Part model, mm, in its own coordinate system. Face numbers are marked on the shaded views. A direction names the side the tool comes from. Round coordinates to 2 decimals unless told otherwise and drop trailing zeros. Order: outer loops, then holes, each group sorted by start corner. A loop starts at its lowest first (then second) coordinate and runs counter-clockwise, first axis right, second up. Notation, with made-up numbers: (61, 87) -> (71, 87) arc R16 cw to (71, 101) -> close; hole circle Ø7 at (-37, 51.25). An arc over 180 degrees is marked (long way). Return JSON: item names as keys, results as strings. Group by question number.
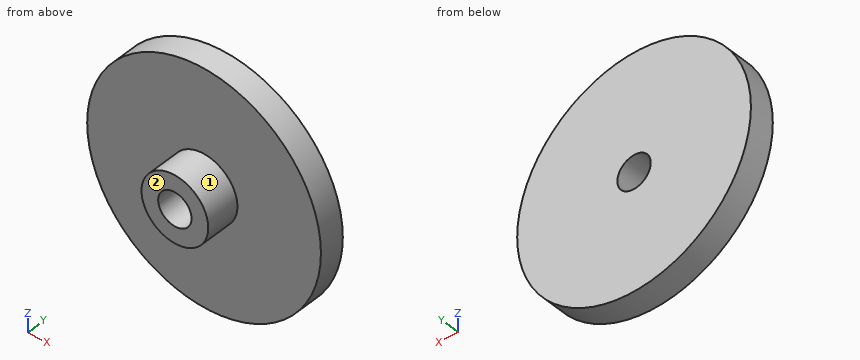
from build123d import *

# Parameters (mm, degrees)
F0_R          = 22.225
F1_DEPTH      = 4.7625
F2_R          = 6.35
F3_DEPTH      = 6.35
F4_R          = 3.175
F5_DEPTH      = 25.4
F5_DEPTH_BACK = 73


# Not quite as in the source:
# - an extrude ends at something that could not be found from the text; its depth is read off the source's solid


with BuildPart() as f1:
    # F0 (on Front) → F1 (new body)
    with BuildSketch(Plane.XZ):
        Circle(F0_R)
    extrude(amount=F1_DEPTH)

    # F2 (on face) → F3 (join)
    with BuildSketch(Plane.XZ.offset(4.7625)):
        Circle(F2_R)
    extrude(amount=F3_DEPTH)

    # F4 (on face) → F5 (cut, two sides)
    with BuildSketch(Plane.XZ.offset(11.1125)) as f5_sk:
        Circle(F4_R)
    extrude(amount=-F5_DEPTH, mode=Mode.SUBTRACT)
    extrude(f5_sk.sketch, amount=F5_DEPTH_BACK, mode=Mode.SUBTRACT)


solid = f1.part
(1) Tool access for the marked faces 1 and 2: list every direction of +Z, -Z, +X, -X, +Y, -Y with a clear straight run to the whole face (end or side of a thin tool).
(2) Saw through at D-D, the plane z = -7.5. List the corners of the cut face in (x, y).
(3) Pin check, flat tips, straight feed: P1, Ø1, axis at x = 4, z = 16, coming from the -Y side; P2, Ø4, axis at x = -14, y = -6.5, coming from the +Z side; P3, Ø2, axis at y = -3.5, z = 15.5, coming from the -X side. Stop position of each tip, or through.
(4) Saw through at C-C, the plane y = -5.5. List the corners of the cut face in (x, z) (3 decimals).
(5) Probe L1, parallel to Z at x = 0, y = -3 (3 decimals); L2, parallel to Z at x = 0, y = -5.25 (3 decimals); L3, parallel to Y at x = 5.5, z = 18. List the from-to ranges inside material, lowest first. Write a range as [from, to].
Results are:
{
 "1": {"face 1": "-Y", "face 2": "+Z, -Z, +X, -X, -Y"},
 "2": {"outline": "(-20.92, -4.76) -> (20.92, -4.76) -> (20.92, 0) -> (-20.92, 0) -> close"},
 "3": {"P1": "stops at y = -4.76", "P2": "stops at z = 18.02", "P3": "stops at x = -16.84"},
 "4": {"outline": "circle Ø12.7 at (0, 0); hole circle Ø6.35 at (0, 0)"},
 "5": {"L1": "z = [-22.225, -3.175], [3.175, 22.225]", "L2": "z = [-6.35, -3.175], [3.175, 6.35]", "L3": "y = [-4.76, 0]"}
}
